from build123d import *

# Parameters (mm, degrees)
F1_DEPTH      = 254
F1_DEPTH_BACK = 254


with BuildPart() as f1:
    # F0 (on Front) → F1 (new body, two sides)
    with BuildSketch(Plane.XZ) as f1_sk:
        with BuildLine():
            Line((6.35, 222.25), (0, 215.9))
            Line((0, 215.9), (0, 86.396878))
            Line((0, 86.396878), (58.90925, 25.394564))
            Line((58.90925, 25.394564), (58.543826, 25.041678))
            Line((58.543826, 25.041678), (81.790096, 0.96946))
            ThreePointArc((81.790096, 0.96946), (84.074, 0), (86.357904, 0.96946))
            Line((86.357904, 0.96946), (101.649771, 16.804652))
            Line((101.649771, 16.804652), (44.45, 127))
            ThreePointArc((44.45, 127), (42.545992, 149.479528), (57.15, 166.6748))
            Line((57.15, 166.6748), (111.125, 180.975))
            Line((111.125, 180.975), (111.125, 222.25))
            Line((111.125, 222.25), (88.138, 222.25))
            Line((88.138, 222.25), (88.138, 238.125))
            Line((88.138, 238.125), (75.438, 238.125))
            Line((75.438, 238.125), (75.438, 222.25))
            Line((75.438, 222.25), (6.35, 222.25))
        make_face()
    extrude(amount=F1_DEPTH)
    extrude(f1_sk.sketch, amount=-F1_DEPTH_BACK)


solid = f1.part
Design review of the part built by this model. Coordinates are the model's own, in mm. A direction names the side the tool comes from. Give positions to 0.01 mm unless a question says otherwise; leave off trailing zeros. Loops run counter-clockwise (first coordinate to the right, second up) from the corner with the lowest first, then second, coordinate; pieces in that order, holes last. Notation, with made-up numbers: (-17.75, -29.75) -> (6.25, -29.75) arc R27 cw to (6.25, -1.75) -> close; hole circle Ø10 at (3, 40). An arc over 180 degrees is marked (long way). One line per question, with ' | ' between items. Start each with the question number.
(1) For line 1 (X direction, y = 175, z = 141); line 2 (Z direction, x = 40.5, y = -170); line 3 (Z direction, x = 76.5, y = 23) (3 decimals), list the stretches that pass through material, from the lowest coordinate up.
(2) We need section D-D (x = 14.5). State the section outline as (y, z) points, and give its area (3 significant figures).
(3) Draft analysis for pull direction Z (two halves, no side actions). For faces 1 (the face through (41, -4, 222.25)), 2 (the face through (0, -4, 152)), 3 (the face through (70.004, -3.556, 13.174)), 4 (the face through (42.45, -3.56, 149.17)), state which applies: +Z half, -Z half, draft (parallel to the pull), parting line (faces both ways), or undercut.
(4) We need section A-A (y = -7). State the section outline as (x, z) points (3 decimals), and give its area (3 significant figures).
(5) For faces 5 (the face through (73.45, -3.56, 71.13)), 6 (the face through (82, -4, 238.125)), 7 (the face through (100, -4, 222.25)), 8 (the face through (75.438, -4, 230)), list the 3-axis set-ups (+Z, -Z, +X, -X, +Y, -Y) from which the entire face can be reached by the end or side of a thin tool; tool diameter is ignored.
(6) Insertion check: P1, Ø17.5, axis at y = 84, z = 228, coming from the -X side; P2, Ø6, axis at x = 22, y = -133.5, coming from the +Z side; P3, Ø8, axis at y = -28.5, z = 232.5, coming from the +X side. Each pin has a flat end and moves straight along its axis. Give the tip position at first contact, or say it passes through.
(7) We need section B-B (x = 94.5). State the section outline as (y, z) points.
(8) We need section C-C (z = 35.5). State the section outline as (x, y) points.
The answers:
1) line 1: x = 0 to 41.15 | line 2: z = 44.46 to 222.25 | line 3: z = 6.448 to 65.256, 171.801 to 238.125
2) outline: (-254, 71.38) -> (254, 71.38) -> (254, 222.25) -> (-254, 222.25) -> close | area: 76,600 mm^2
3) face 1: +Z half | face 2: draft | face 3: -Z half | face 4: undercut
4) outline: (0, 86.397) -> (58.909, 25.395) -> (58.544, 25.042) -> (81.79, 0.969) arc R3.175 ccw to (86.358, 0.969) -> (101.65, 16.805) -> (44.45, 127) arc R29.363 cw to (57.15, 166.675) -> (111.125, 180.975) -> (111.125, 222.25) -> (88.138, 222.25) -> (88.138, 238.125) -> (75.438, 238.125) -> (75.438, 222.25) -> (6.35, 222.25) -> (0, 215.9) -> close | area: 13,800 mm^2
5) face 5: +X, +Y, -Y | face 6: +Z, +X, -X, +Y, -Y | face 7: +Z, +X, +Y, -Y | face 8: +Z, -X, +Y, -Y
6) P1: stops at x = 3.35 | P2: stops at z = 222.25 | P3: stops at x = 88.14
7) outline: (-254, 9.4) -> (254, 9.4) -> (254, 30.58) -> (-254, 30.58) -> close; (-254, 176.57) -> (254, 176.57) -> (254, 222.25) -> (-254, 222.25) -> close
8) outline: (49.15, -254) -> (91.95, -254) -> (91.95, 254) -> (49.15, 254) -> close
